Design review of the part built by this model. Coordinates are the model's own, in mm. A direction names the side the tool comes from. Round coordinates to 2 decimals unless told otherwise and drop trailing zeros. Write each loop counter-clockwise with the first axis right and the second up, starting at its lowest first coordinate (ties: lowest second). Pieces come first, ordered by that corner, then holes. Notation, with made-up numbers: (81.25, 61.25) -> (113.25, 61.25) arc R17 ccw to (113.25, 86.25) -> close; hole circle Ø11 at (68.5, 52). An arc over 180 degrees is marked (long way). Write item = value, one per line. Start each with the question number.
Item 1: For pin 1 Ø12 at (y, z) = (15, -20) entering from +X; pin 2 Ø5 at (x, z) = (-9, 7) entering from -Y; pin 3 Ø6 at (y, z) = (10.5, 2) entering from -X; pin 4 Ø2.5 at (x, y) = (24.15, 5) entering from +Z, all flat-tipped, find the tip position at first contact; note any pin that passes through.
Item 2: Machinability: for faces 1 (the cylindrical face through (-2.02, 10.99, -26.77)), 2 (the flat face through (-24, 10, -7.7)), 3 (the flat face through (20.15, 10, 6)), 4 (the cylindrical face through (-5.518, 6.448, -22.458)), which of the approach directions +Z, -Z, +X, -X, +Y, -Y give a long, thin tool a straight path to every point of the face, cutting with its end or side? Answer none if there is none.
Item 3: Add section D-D, the plane y = 18. State the section outline as (x, z) points, then the cut area to 3 significant figures.
Item 4: Add section C-C, the plane x = 8. State the section outline as (y, z) points.
Item 5: Add section A-A, the plane x = -24.15. State the section outline as (y, z) points.
Item 6: Add section B-B, the plane y = 10. State the section outline as (x, z) points, then the cut area to 3 significant figures.
Item 7: Mouldability with a two-part tool opening along X and no side actions: class faces 5 (the flat face through (27.25, 10, -9)), 6 (the flat face through (0, 0, 0)), 7 (the cylindrical face through (-9.15, 2.04, -26.77)), 8 (the cylindrical face through (-19.104, 10.3, -26.768)) as released by +X, released by -X, zero draft, split by the parting line, or undercut.
Item 8: To check wall thickness, follow L1, parallel to Y at x = -24, z = -9; L2, parallel to Z at x = -16, y = 17; L3, parallel to X at y = 10, z = -6.5. State the ranges of each line that lie inside material, in increasing order.
from build123d import *

# Parameters (mm, degrees)
SALIENTE_EXTRUIR1_DEPTH = 20
CROQUIS3_R              = 5.837463161
SALIENTE_EXTRUIR3_DEPTH = 8.5
CROQUIS4_R              = 2
CORTAR_EXTRUIR1_DEPTH   = 10
CROQUIS5_R              = 10.5
SALIENTE_EXTRUIR4_DEPTH = 2.5
CORTAR_EXTRUIR3_REACH   = 49.5
CROQUIS6_R              = 1


with BuildPart() as part:
    # Croquis1 → Saliente-Extruir1 (new body)
    with BuildSketch(Plane(origin=(0, 0, 0), x_dir=(1, 0, 0), z_dir=(0, 1, 0))):
        Polygon((20.15, 19.5), (-20.15, 19.5), (-20.15, 10.5), (-27.25, 10.5), (-27.25, 7.7), (-20.15, 7.7), (-20.15, -19.5), (20.15, -19.5), (20.15, 7.7), (27.25, 7.7), (27.25, 10.5), (20.15, 10.5), align=None)
    extrude(amount=SALIENTE_EXTRUIR1_DEPTH)

    # Croquis3 → Saliente-Extruir3 (add)
    with BuildSketch(Plane(origin=(0, 0, -19.5), x_dir=(-1, 0, 0), z_dir=(0, 0, -1))):
        with Locations((10.15, 10)):
            Circle(CROQUIS3_R)
    extrude(amount=SALIENTE_EXTRUIR3_DEPTH)

    # Croquis4 → Cortar-Extruir1 (cut)
    with BuildSketch(Plane(origin=(0, 0, -10.5), x_dir=(-1, 0, 0), z_dir=(0, 0, -1))):
        with Locations((-24.15, 15)):
            Circle(CROQUIS4_R)
        with Locations((-24.15, 5)):
            Circle(CROQUIS4_R)
        with Locations((24.15, 5)):
            Circle(CROQUIS4_R)
        with Locations((24.15, 15)):
            Circle(CROQUIS4_R)
    extrude(amount=-CORTAR_EXTRUIR1_DEPTH, mode=Mode.SUBTRACT)

    # Croquis5 → Saliente-Extruir4 (add)
    with BuildSketch(Plane(origin=(0, 0, -28), x_dir=(-1, 0, 0), z_dir=(0, 0, -1))):
        with Locations((10.15, 10)):
            Circle(CROQUIS5_R)
    extrude(amount=-SALIENTE_EXTRUIR4_DEPTH)

    # Croquis6 → Cortar-Extruir3 (cut, up to next)
    with BuildSketch(Plane(origin=(0, 0, -28), x_dir=(-1, 0, 0), z_dir=(0, 0, -1)), mode=Mode.PRIVATE) as cortar_extruir3_sk1:
        with Locations((10.15, 18)):
            Circle(CROQUIS6_R)
    cortar_extruir3_tool1 = extrude(cortar_extruir3_sk1.sketch, amount=-CORTAR_EXTRUIR3_REACH, mode=Mode.PRIVATE) & part.part
    add(cortar_extruir3_tool1.solids().sort_by_distance((-10.15, 18, -28))[0], mode=Mode.SUBTRACT)
    # Croquis6 → Cortar-Extruir3 (cut, up to next)
    with BuildSketch(Plane(origin=(0, 0, -28), x_dir=(-1, 0, 0), z_dir=(0, 0, -1)), mode=Mode.PRIVATE) as cortar_extruir3_sk2:
        with Locations((18.15, 10)):
            Circle(CROQUIS6_R)
    cortar_extruir3_tool2 = extrude(cortar_extruir3_sk2.sketch, amount=-CORTAR_EXTRUIR3_REACH, mode=Mode.PRIVATE) & part.part
    add(cortar_extruir3_tool2.solids().sort_by_distance((-18.15, 10, -28))[0], mode=Mode.SUBTRACT)
    # Croquis6 → Cortar-Extruir3 (cut, up to next)
    with BuildSketch(Plane(origin=(0, 0, -28), x_dir=(-1, 0, 0), z_dir=(0, 0, -1)), mode=Mode.PRIVATE) as cortar_extruir3_sk3:
        with Locations((2.15, 10)):
            Circle(CROQUIS6_R)
    cortar_extruir3_tool3 = extrude(cortar_extruir3_sk3.sketch, amount=-CORTAR_EXTRUIR3_REACH, mode=Mode.PRIVATE) & part.part
    add(cortar_extruir3_tool3.solids().sort_by_distance((-2.15, 10, -28))[0], mode=Mode.SUBTRACT)
    # Croquis6 → Cortar-Extruir3 (cut, up to next)
    with BuildSketch(Plane(origin=(0, 0, -28), x_dir=(-1, 0, 0), z_dir=(0, 0, -1)), mode=Mode.PRIVATE) as cortar_extruir3_sk4:
        with Locations((10.15, 2)):
            Circle(CROQUIS6_R)
    cortar_extruir3_tool4 = extrude(cortar_extruir3_sk4.sketch, amount=-CORTAR_EXTRUIR3_REACH, mode=Mode.PRIVATE) & part.part
    add(cortar_extruir3_tool4.solids().sort_by_distance((-10.15, 2, -28))[0], mode=Mode.SUBTRACT)


solid = part.part
Result set:
q1.pin_1 = 20.15
q1.pin_2 = 0
q1.pin_3 = -20.15
q1.pin_4 = through
q2.face_1 = -Z
q2.face_2 = +Z, -X, +Y, -Y
q2.face_3 = +Z, +X, +Y, -Y
q2.face_4 = none
q3.outline = (-27.25, -10.5) -> (-20.15, -10.5) -> (-20.15, -19.5) -> (20.15, -19.5) -> (20.15, -10.5) -> (27.25, -10.5) -> (27.25, -7.7) -> (20.15, -7.7) -> (20.15, 19.5) -> (-20.15, 19.5) -> (-20.15, -7.7) -> (-27.25, -7.7) -> close; (-16.95, -28) -> (-11.15, -28) -> (-11.15, -25.5) -> (-16.95, -25.5) -> close; (-9.15, -28) -> (-3.35, -28) -> (-3.35, -25.5) -> (-9.15, -25.5) -> close
q3.area = 1,640 mm²
q4.outline = (0, -19.5) -> (20, -19.5) -> (20, 19.5) -> (0, 19.5) -> close
q5.outline = (0, -10.5) -> (3, -10.5) -> (3, -7.7) -> (0, -7.7) -> close; (7, -10.5) -> (13, -10.5) -> (13, -7.7) -> (7, -7.7) -> close; (17, -10.5) -> (20, -10.5) -> (20, -7.7) -> (17, -7.7) -> close
q6.outline = (-27.25, -10.5) -> (-20.15, -10.5) -> (-20.15, -19.5) -> (-15.99, -19.5) -> (-15.99, -25.5) -> (-17.15, -25.5) -> (-17.15, -28) -> (-3.15, -28) -> (-3.15, -25.5) -> (-4.31, -25.5) -> (-4.31, -19.5) -> (20.15, -19.5) -> (20.15, -10.5) -> (27.25, -10.5) -> (27.25, -7.7) -> (20.15, -7.7) -> (20.15, 19.5) -> (-20.15, 19.5) -> (-20.15, -7.7) -> (-27.25, -7.7) -> close; (-20.65, -28) -> (-19.15, -28) -> (-19.15, -25.5) -> (-20.65, -25.5) -> close; (-1.15, -28) -> (0.35, -28) -> (0.35, -25.5) -> (-1.15, -25.5) -> close
q6.area = 1,720 mm²
q7.face_5 = released by +X
q7.face_6 = zero draft
q7.face_7 = undercut
q7.face_8 = undercut
q8.L1 = 0 to 3.01, 6.99 to 13.01, 16.99 to 20
q8.L2 = -28 to -25.5, -19.5 to 19.5
q8.L3 = -20.15 to 20.15
